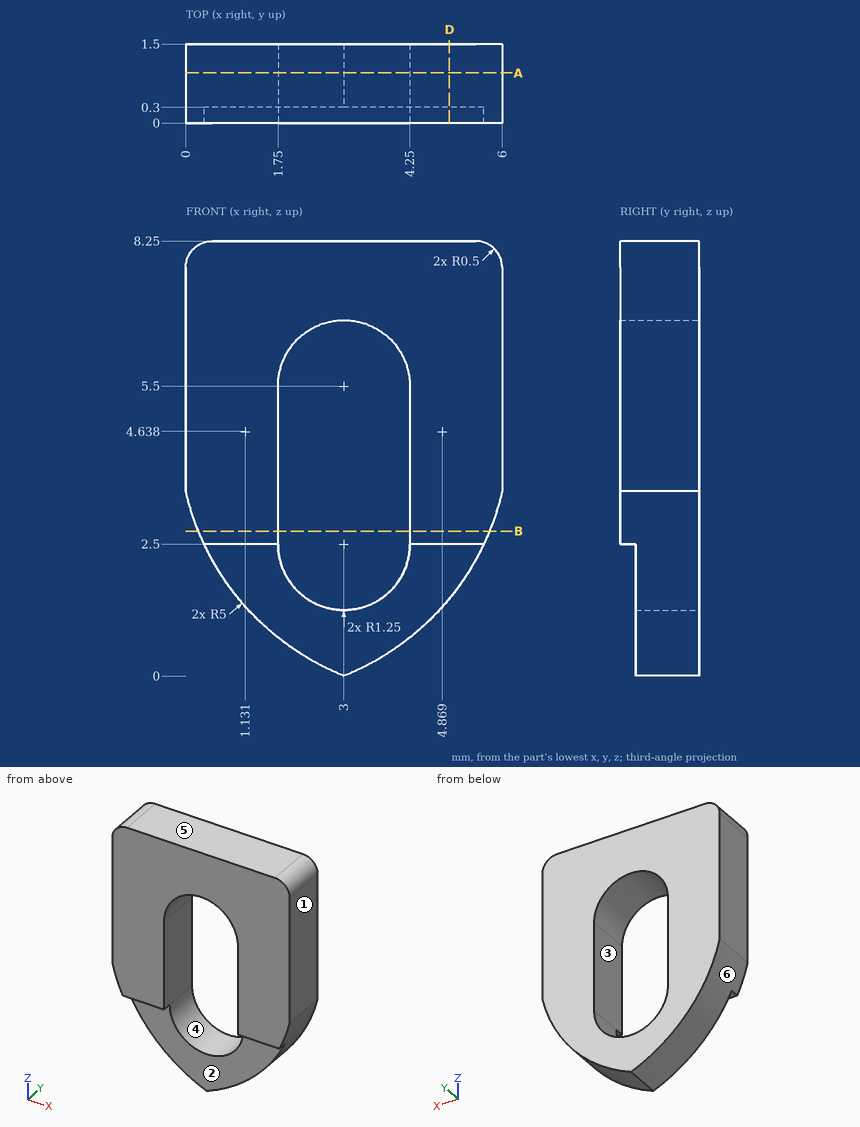
Answer from the drawing. Dimensions are ordinates in mm from the lowest x, y and z of the part. A direction names the side the tool comes from. Give positions to 0.01 mm unless a question says otherwise; leave off trailing zeros. Loops run counter-clockwise (first coordinate to the right, second up) from the corner with the lowest first, then second, coordinate; pieces in that order, holes last.
Item 1: Find the intervals of material crossed by line 1 along X through (y, z) = (0.55, 4.25); line 2 along X through (y, z) = (1.2, 2.5); line 3 along Z through (x, y) = (2.25, 1.3), in increasing order.
Item 2: The part is cut by section D-D (x = 5). Write down the section's boundary in (y, z).
Item 3: The part is cut by section B-B (z = 2.75). Write down the section's boundary in (x, y).
Item 4: This flat-tipped pin is pushed along its axis until it touches: pin 1 Ø1.3 at (x, z) = (2.5, 1.5) entering from -Y. Where does it stop, or does it pass through?
Item 5: The mould has two halves that part along Z. Classify the marked faces 4, 5 and 6: released by +Z, released by -Z, zero draft, split by the parting line, or undercut.
Item 6: The part is cut by section A-A (y = 0.95). Write down the section's boundary in (x, z).
Item 7: For the marked faces 1, 2 and 3, determine the directions among +Z, -Z, +X, -X, +Y, -Y from which every point of the face is accessible in a straight line to the end or side of a thin tool.
Taken from the geometry:
1. line 1: x = 0 to 1.75, 4.25 to 6
1. line 2: x = 0.35 to 1.75, 4.25 to 5.65
1. line 3: z = 0.38 to 1.5, 6.5 to 8.25
2. outline: (0, 2.5) - (0.3, 2.5) - (0.3, 1.47) - (1.5, 1.47) - (1.5, 8.25) - (0, 8.25) - close
3. outline: (0.24, 0) - (1.75, 0) - (1.75, 1.5) - (0.24, 1.5) - close; (4.25, 0) - (5.76, 0) - (5.76, 1.5) - (4.25, 1.5) - close
4. pin 1: stops at y = 0.3
5. face 4: undercut
5. face 5: released by +Z
5. face 6: released by -Z
6. outline: (0, 3.5) arc R5 ccw to (3, 0) arc R5 ccw to (6, 3.5) - (6, 7.75) arc R0.5 ccw to (5.5, 8.25) - (0.5, 8.25) arc R0.5 ccw to (0, 7.75) - close; hole (1.75, 2.5) arc R1.25 ccw to (4.25, 2.5) - (4.25, 5.5) arc R1.25 ccw to (1.75, 5.5) - close
7. face 1: +Z, -Z, +X, +Y, -Y
7. face 2: -Z, +X, -X, -Y
7. face 3: +Y, -Y
